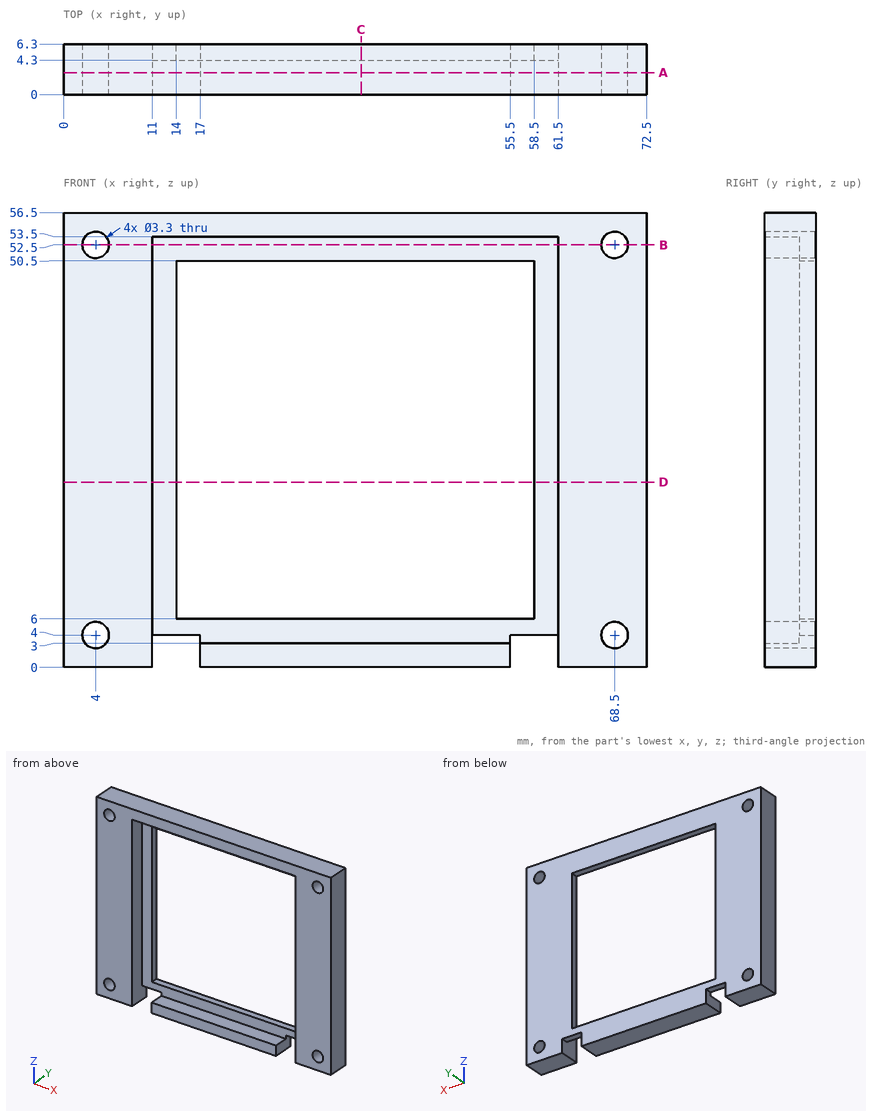
For this review, use the dimensioned drawing (mm, ordinates from the lowest corner) and the shaded views. Give positions to 0.01 mm unless a question says otherwise; leave off trailing zeros. Order: outer loops, then holes, each group sorted by start corner. A loop starts at its lowest first (then second) coordinate and runs counter-clockwise, first axis right, second up. Notation, with made-up numbers: (75.25, -5.5) - (89.25, -5.5) arc R10 cw to (89.25, 12.5) - close; hole circle Ø2 at (87.25, -39.5). An arc over 180 degrees is marked (long way). Use a Markdown table: item, result. Add a question column.
(1) Add section C-C on x = 37. Give the boundary of the cut face in (y, z), then the cut area to 3 significant figures.
(2) Clearance check with flat-ended pins moving along their axes: P1, Ø2.5, axis at x = 4, z = 52.5, coming from the -Y side; P2, Ø1, axis at x = 13.5, y = 5.5, coming from the -Z side. State where each tip first meets the part, or that it passes through.
(3) Add section B-B on z = 52.5. Give the boundary of the cut face in (x, y), then the cut area to 3 significant figures.
(4) Add section A-A on y = 2.75. Give the boundary of the cut face in (x, z), then the cut area to 3 significant figures.
(5) Add section D-D on z = 23. Give the boundary of the cut face in (x, y).
(6) Wall thickness on probe 1 along X at (y, z) = (3, 52.5); probe 2 along Z at (x, y) = (4, 2.25); probe 3 along X at (y, z) = (4.5, 52.5): over which ranges is each line inside the solid? List them lowest first. Write a range as [from, to].
Report:
| question | item | result |
|---|---|---|
| 1 | outline | (0, 0) - (6.3, 0) - (6.3, 6) - (4.3, 6) - (4.3, 3) - (0, 3) - close; (0, 53.5) - (4.3, 53.5) - (4.3, 50.5) - (6.3, 50.5) - (6.3, 56.5) - (0, 56.5) - close |
| 1 | area | 49.8 mm² |
| 2 | P1 | passes through |
| 2 | P2 | stops at z = 4 |
| 3 | outline | (0, 0) - (2.35, 0) - (2.35, 6.3) - (0, 6.3) - close; (5.65, 0) - (11, 0) - (11, 4.3) - (61.5, 4.3) - (61.5, 0) - (66.85, 0) - (66.85, 6.3) - (5.65, 6.3) - close; (70.15, 0) - (72.5, 0) - (72.5, 6.3) - (70.15, 6.3) - close |
| 3 | area | 198 mm² |
| 4 | outline | (0, 0) - (11, 0) - (11, 53.5) - (61.5, 53.5) - (61.5, 0) - (72.5, 0) - (72.5, 56.5) - (0, 56.5) - close; (17, 0) - (55.5, 0) - (55.5, 3) - (17, 3) - close; hole circle Ø3.3 at (4, 4); hole circle Ø3.3 at (4, 52.5); hole circle Ø3.3 at (68.5, 4); hole circle Ø3.3 at (68.5, 52.5) |
| 4 | area | 1,480 mm² |
| 5 | outline | (0, 0) - (11, 0) - (11, 4.3) - (14, 4.3) - (14, 6.3) - (0, 6.3) - close; (58.5, 4.3) - (61.5, 4.3) - (61.5, 0) - (72.5, 0) - (72.5, 6.3) - (58.5, 6.3) - close |
| 6 | probe 1 | x = [0, 2.35], [5.65, 11], [61.5, 66.85], [70.15, 72.5] |
| 6 | probe 2 | z = [0, 2.35], [5.65, 50.85], [54.15, 56.5] |
| 6 | probe 3 | x = [0, 2.35], [5.65, 66.85], [70.15, 72.5] |
